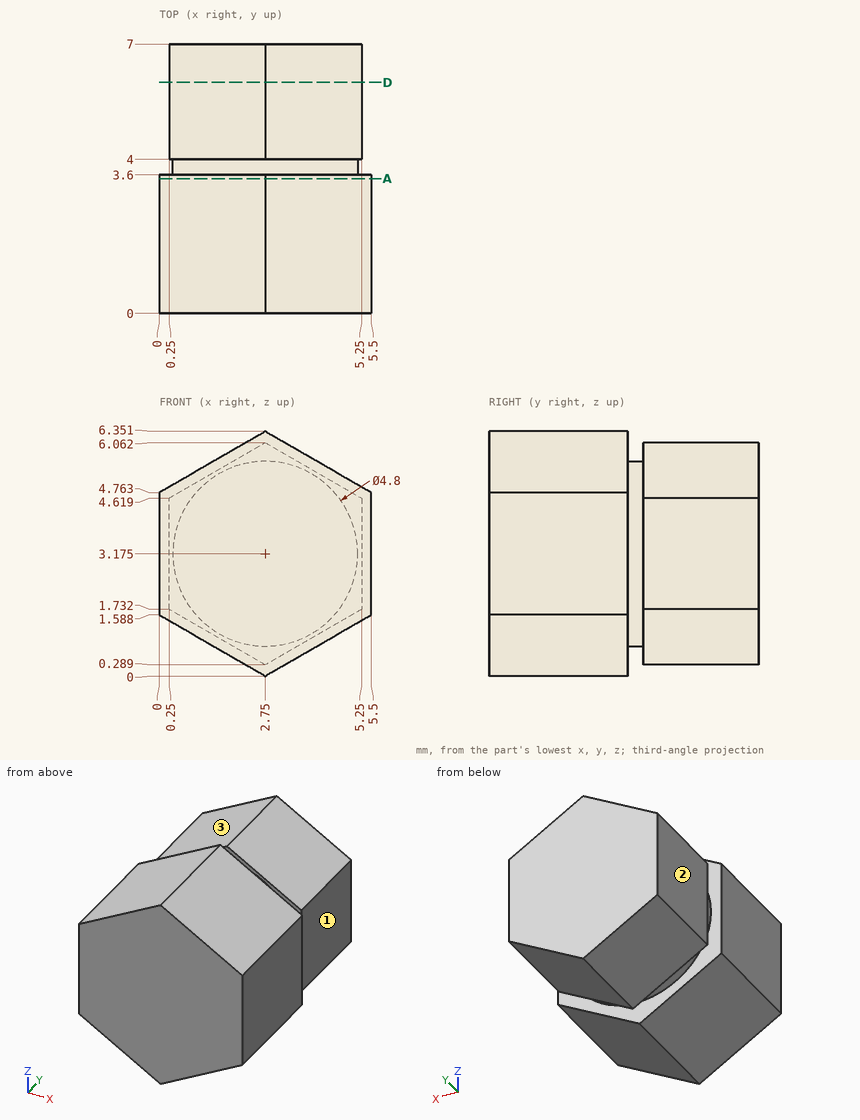
Check sheet for the drawn part. Datum: minimum x, y, z corner. Units: mm. A direction names the side the tool comes from. Round coordinates to 2 decimals unless told otherwise and drop trailing zeros. Order: outer loops, then holes, each group sorted by start corner. A loop starts at its lowest first (then second) coordinate and runs counter-clockwise, first axis right, second up.
1. Section check A-A on y = 3.5. Record the cut outline in (x, z), then the cut area to 3 significant figures.
Final values:
outline: (0, 1.59) - (2.75, 0) - (5.5, 1.59) - (5.5, 4.76) - (2.75, 6.35) - (0, 4.76) - close
area: 26.2 mm2
2. Go/stop test with flat-tipped pins: P1, Ø1.5, axis at x = 2.5, z = 3, coming from the -Y side; P2, Ø1.4, axis at y = 5, z = 3, coming from the -X side. Record where each tip stops, or that it passes through.
Final values:
P1: stops at y = 0
P2: stops at x = 0.25
3. Thickness scan on L1, parallel to X at y = 5.25, z = 2; L2, parallel to Y at x = 0.2, z = 4.25; L3, parallel to X at y = 6.75, z = 5.25 (1 decimal). Record the ranges inside material, lowest first.
Final values:
L1: x = 0.25 to 5.25
L2: y = 0 to 3.6
L3: x = 1.3 to 4.2
4. Section check D-D on y = 6. Record the cut outline in (x, z).
Final values:
outline: (0.25, 1.73) - (2.75, 0.29) - (5.25, 1.73) - (5.25, 4.62) - (2.75, 6.06) - (0.25, 4.62) - close
5. Access from +Z, -Z, +X, -X, +Y, -Y to the whole of each face (thin tool, end or side, straight path). Record for the marked faces 1, 2 and 3.
Final values:
face 1: +Z, -Z, +X, +Y
face 2: +Z, -Z, -X, +Y
face 3: +Z, -X, +Y
